For this review, take the finished solid that the model builds, in its own axes (mm). Coordinates: 2 decimals unless noted, no trailing zeros. Order: outer loops, then holes, each group sorted by start corner. A loop starts at its lowest first (then second) coordinate and runs counter-clockwise, first axis right, second up. Notation, with made-up numbers: (-36, 32) -> (-10, 32) arc R20 cw to (-10, 56) -> close; hole circle Ø7 at (33, -11). An arc over 180 degrees is marked (long way). Write item = value, one per line. Start each with the question number.
1) Consider section D-D on y = 14. Give the boundary of the cut face in (x, z).
2) Consider section A-A on y = 0. Give the boundary of the cut face in (x, z), and give its area (3 significant figures).
3) Insertion check: pin 1 Ø4 at (x, z) = (-34, 8.5) entering from -Y; pin 2 Ø5 at (x, z) = (-139, 3) entering from +Y; pin 3 Ø3 at (x, z) = (-42, 8.5) entering from +Y; pin 4 Ø24 at (x, y) = (0, 0) entering from +Z. Each pin has a flat end and moves straight along its axis. Give the tip position at first contact, or say it passes through.
4) Wall thickness on probe 1 along Y at (x, z) = (30, 6.25); probe 2 along Y at (x, z) = (8, 7); probe 3 along X at (y, z) = (-11.5, 7.25): over which ranges is each line inside the solid? List them lowest first. Write a range as [from, to].
5) Consider section B-B on z = 8.25. Give the boundary of the cut face in (x, y).
6) Consider section C-C on x = 0. Give the boundary of the cut face in (y, z), and give its area (3 significant figures).
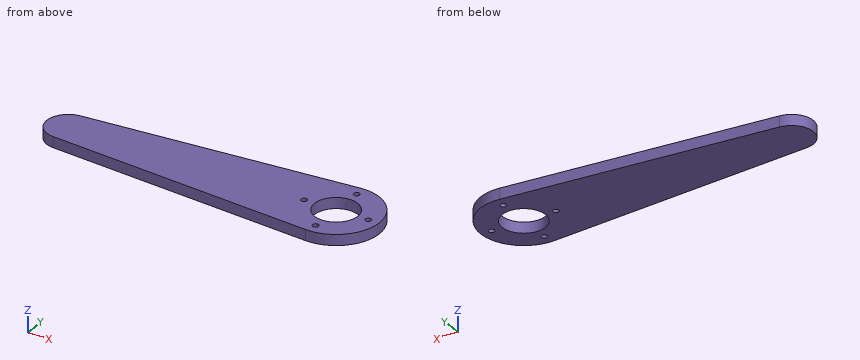
from build123d import *

# Parameters (mm, degrees)
SKETCH_R           = 20
PAD_DEPTH          = 10
SKETCH001_R        = 2.75
HOLE_DEPTH         = 25
POLARPATTERN_COUNT = 4


with BuildPart() as part:
    # Sketch → Pad (new body)
    with BuildSketch(Plane.XY):
        with BuildLine():
            ThreePointArc((-251.6, 19.935897), (-270, 0), (-251.6, -19.935897))
            Line((-251.6, -19.935897), (-3.2, -39.871795))
            ThreePointArc((-3.2, -39.871795), (40, 0), (-3.2, 39.871795))
            Line((-251.6, 19.935897), (-3.2, 39.871795))
        make_face()
        Circle(SKETCH_R, mode=Mode.SUBTRACT)
    extrude(amount=PAD_DEPTH)

    # Sketch001 (on Face7 of Pad) → Hole (cut)
    with BuildSketch(Plane.XY.offset(10)):
        with Locations((30, 0)):
            Circle(SKETCH001_R)
    hole = extrude(amount=-HOLE_DEPTH, mode=Mode.SUBTRACT)

    # PolarPattern: Hole ×4 about axis
    polarpattern_axis = Axis((0, 0, 10), (0, 0, 1))
    for i in range(1, POLARPATTERN_COUNT):
        add(hole.rotate(polarpattern_axis, i * 360 / POLARPATTERN_COUNT), mode=Mode.SUBTRACT)


solid = part.part
Answer sheet:
q1.outline = (-264.28, 0) -> (-14.28, 0) -> (-14.28, 10) -> (-264.28, 10) -> close; (14.28, 0) -> (37.47, 0) -> (37.47, 10) -> (14.28, 10) -> close
q2.outline = (-270, 0) -> (-32.75, 0) -> (-32.75, 10) -> (-270, 10) -> close; (-27.25, 0) -> (-20, 0) -> (-20, 10) -> (-27.25, 10) -> close; (20, 0) -> (27.25, 0) -> (27.25, 10) -> (20, 10) -> close; (32.75, 0) -> (40, 0) -> (40, 10) -> (32.75, 10) -> close
q2.area = 2,590 mm2
q3.pin_1 = -37.56
q3.pin_2 = 29.17
q3.pin_3 = 36.88
q3.pin_4 = through
q4.probe_1 = [-26.46, -2.75], [2.75, 26.46]
q4.probe_2 = [-39.19, -18.33], [18.33, 39.19]
q4.probe_3 = [-266.36, -16.36], [16.36, 38.31]
q5.outline = (-251.6, -19.94) -> (-3.2, -39.87) arc R40 ccw (long way) to (-3.2, 39.87) -> (-251.6, 19.94) arc R20 ccw to start; hole circle Ø5.5 at (-30, 0); hole circle Ø40 at (0, 0); hole circle Ø5.5 at (0, -30); hole circle Ø5.5 at (0, 30); hole circle Ø5.5 at (30, 0)
q6.outline = (-40, 0) -> (-32.75, 0) -> (-32.75, 10) -> (-40, 10) -> close; (-27.25, 0) -> (-20, 0) -> (-20, 10) -> (-27.25, 10) -> close; (20, 0) -> (27.25, 0) -> (27.25, 10) -> (20, 10) -> close; (32.75, 0) -> (40, 0) -> (40, 10) -> (32.75, 10) -> close
q6.area = 290 mm2
